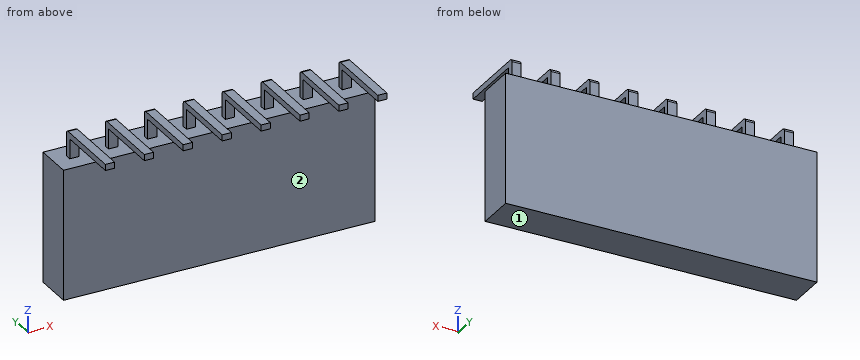
from build123d import *

# Parameters (mm, degrees)
SKETCH_1_W      = 20.32
SKETCH_1_H      = 8.5
EXTRUDE_1_DEPTH = 2.5
SKETCH_2_W      = 0.6
SKETCH_2_H      = 0.4
EXTRUDE_2_DEPTH = 1.7
SKETCH_3_W      = 0.6
SKETCH_3_H      = 0.4
EXTRUDE_3_DEPTH = 4.35
FILLET_1_R      = 0.2


with BuildPart() as part:
    # Эскиз1 → Бобышка-Вытянуть1 (new body)
    with BuildSketch(Plane(origin=(0, 0, 0), x_dir=(1, 0, 0), z_dir=(0, 1, 0))):
        Rectangle(SKETCH_1_W, SKETCH_1_H)
    extrude(amount=EXTRUDE_1_DEPTH)

    # Эскиз2 → Бобышка-Вытянуть2 (add)
    with BuildSketch(Plane.XY.offset(4.25)):
        with Locations((-6.35, 1.25)):
            Rectangle(SKETCH_2_W, SKETCH_2_H)
        with Locations((-8.89, 1.25)):
            Rectangle(SKETCH_2_W, SKETCH_2_H)
        with Locations((-3.81, 1.25)):
            Rectangle(SKETCH_2_W, SKETCH_2_H)
        with Locations((-1.27, 1.25)):
            Rectangle(SKETCH_2_W, SKETCH_2_H)
        with Locations((1.27, 1.25)):
            Rectangle(SKETCH_2_W, SKETCH_2_H)
        with Locations((3.81, 1.25)):
            Rectangle(SKETCH_2_W, SKETCH_2_H)
        with Locations((6.35, 1.25)):
            Rectangle(SKETCH_2_W, SKETCH_2_H)
        with Locations((8.89, 1.25)):
            Rectangle(SKETCH_2_W, SKETCH_2_H)
    extrude(amount=EXTRUDE_2_DEPTH)

    # Эскиз3 → Бобышка-Вытянуть3 (add)
    with BuildSketch(Plane.XZ.offset(-1.05)):
        with Locations((-8.89, 5.75)):
            Rectangle(SKETCH_3_W, SKETCH_3_H)
        with Locations((-6.35, 5.75)):
            Rectangle(SKETCH_3_W, SKETCH_3_H)
        with Locations((-3.81, 5.75)):
            Rectangle(SKETCH_3_W, SKETCH_3_H)
        with Locations((-1.27, 5.75)):
            Rectangle(SKETCH_3_W, SKETCH_3_H)
        with Locations((1.27, 5.75)):
            Rectangle(SKETCH_3_W, SKETCH_3_H)
        with Locations((3.81, 5.75)):
            Rectangle(SKETCH_3_W, SKETCH_3_H)
        with Locations((6.35, 5.75)):
            Rectangle(SKETCH_3_W, SKETCH_3_H)
        with Locations((8.89, 5.75)):
            Rectangle(SKETCH_3_W, SKETCH_3_H)
    extrude(amount=EXTRUDE_3_DEPTH)

    # Скругление1
    fillet_1_edges = [part.edges().sort_by_distance(p)[0] for p in [
        (-8.89, 1.45, 5.95),
        (-6.35, 1.45, 5.95),
        (-3.81, 1.45, 5.95),
        (-1.27, 1.45, 5.95),
        (1.27, 1.45, 5.95),
        (3.81, 1.45, 5.95),
        (6.35, 1.45, 5.95),
        (8.89, 1.45, 5.95),
    ]]
    fillet(fillet_1_edges, radius=FILLET_1_R)


solid = part.part
Verification items for the finished model (mm, model axes). Face numbers are marked on the shaded views. A direction names the side the tool comes from. Give positions to 0.01 mm unless a question says otherwise; leave off trailing zeros. Write each loop counter-clockwise with the first axis right and the second up, starting at its lowest first coordinate (ties: lowest second). Pieces come first, ordered by that corner, then holes. Notation, with made-up numbers: M -20.75,29.25 L -11.75,29.25 A29 ccw -11.75,64.25 Z; hole C 29.25,77.5 d1. An arc over 180 degrees is marked long. Write item = value, one per line.
(1) Sectioned sample at A-A (z = 4.5). Give the number of separate pieces and of enclosed holes in the cut face, then the cut area to 3 significant figures.
Found:
separate_pieces = 8
enclosed_holes = 0
area = 1.92 mm2
(2) Material ranges on line 1 (Z direction, x = -6.25, y = 0.45); line 2 (Y direction, x = -3.25, z = 0.25); line 3 (Z direction, x = -0.5, y = 0.3), recorded low to high.
Found:
line_1 = -4.25 to 4.25, 5.55 to 5.95
line_2 = 0 to 2.5
line_3 = -4.25 to 4.25
(3) Sectioned sample at C-C (x = -2). Record the cut outline in (y, z), then the cut area to 4 significant figures.
Found:
outline = M 0,-4.25 L 2.5,-4.25 L 2.5,4.25 L 0,4.25 Z
area = 21.25 mm2
(4) Sectioned sample at D-D (y = 2.1). Record the cut outline in (x, z), then the cut area to 3 significant figures.
Found:
outline = M -10.16,-4.25 L 10.16,-4.25 L 10.16,4.25 L -10.16,4.25 Z
area = 173 mm2
(5) Go/stop test with flat-tipped pins: pin 1 Ø1.5 at (y, z) = (-1, -0.5) entering from -X; pin 2 Ø1.9 at (y, z) = (-2, 5) entering from +X; pin 3 Ø0.5 at (y, z) = (-1, 5.5) entering from -X; pin 4 Ø0.5 at (x, y) = (-9, -0.5) entering from -Z. Record where each tip stops, or that it passes through.
Found:
pin_1 = through
pin_2 = 9.19
pin_3 = -9.19
pin_4 = 5.55
(6) Access from +Z, -Z, +X, -X, +Y, -Y to the whole of each face (thin tool, end or side, straight path). Record for the marked faces 1 and 2.
Found:
face_1 = -Z, +X, -X, +Y, -Y
face_2 = -Z, +X, -X, -Y
